Could you check a few things on this model? Use its own coordinates, in mm. A direction names the side the tool comes from. Give positions to 0.01 mm unless a question says otherwise; leave off trailing zeros. Loops run counter-clockwise (first coordinate to the right, second up) from the corner with the lowest first, then second, coordinate; pieces in that order, holes last. Notation, with made-up numbers: M -16.75,-33 L 18.25,-33 A24 ccw 18.25,0 Z; hole C 40,5.5 d11. An arc over 180 degrees is marked long. Use CSV: the item, a comma, the result in double quotes.
```python
from build123d import *

# Parameters (mm, degrees)
SKETCH1_W               = 240
SKETCH1_H               = 300
BOSS_EXTRUDE1_DEPTH     = 80
SHELL1_T                = -11
SKETCH4_R               = 1.5
CUT_EXTRUDE2_DEPTH      = 209.086520467
MIRROR2_COPY_1_SKETCH_R = 1.5
MIRROR2_COPY_1_DEPTH    = 209.086520467
SKETCH16_W              = 25
SKETCH16_H              = 8
CUT_EXTRUDE9_DEPTH      = 333.866339542
SKETCH18_W              = 71.1
SKETCH18_H              = 45
SKETCH18_W_2            = 72.7
CUT_EXTRUDE10_DEPTH     = 295.108823397
SKETCH19_W              = 71.1
SKETCH19_H              = 7.810897368
SKETCH19_W_2            = 72.674166019
CUT_EXTRUDE11_DEPTH     = 295.108823397
CUT_EXTRUDE12_DEPTH     = 15


with BuildPart() as part:
    # Sketch1 → Boss-Extrude1 (new body)
    with BuildSketch(Plane(origin=(0, 0, 0), x_dir=(1, 0, 0), z_dir=(0, 1, 0))):
        Rectangle(SKETCH1_W, SKETCH1_H)
    extrude(amount=BOSS_EXTRUDE1_DEPTH)

    # Shell1
    shell1_openings = [part.faces().sort_by_distance(p)[0] for p in [
        (0, 80, 0),
        (0, 0, 0),
    ]]
    offset(amount=SHELL1_T, openings=shell1_openings, kind=Kind.INTERSECTION)

    # Sketch4 → Cut-Extrude2 (cut, through all)
    with BuildSketch(Plane(origin=(0, 80, 0), x_dir=(1, 0, 0), z_dir=(0, 1, 0))):
        with Locations(Location((-112.5, 142.5, 0), (0, 0, 270))):
            Circle(SKETCH4_R)
    cut_extrude2 = extrude(amount=-CUT_EXTRUDE2_DEPTH, mode=Mode.SUBTRACT)

    # Mirror1: Cut-Extrude2 across plane
    add(cut_extrude2.mirror(Plane(origin=(0, 0, 0), x_dir=(0, 0, 1), z_dir=(1, 0, 0))), mode=Mode.SUBTRACT)

    # Mirror2: Cut-Extrude2 across plane
    add(cut_extrude2.mirror(Plane.XY), mode=Mode.SUBTRACT)

    # Mirror2 copy 1 sketch → Mirror2 copy 1 (cut, through all)
    with BuildSketch(Plane(origin=(0, 80, 0), x_dir=(-1, 0, 0), z_dir=(0, 1, 0))):
        with Locations(Location((-112.5, 142.5, 0), (0, 0, 270))):
            Circle(MIRROR2_COPY_1_SKETCH_R)
    extrude(amount=-MIRROR2_COPY_1_DEPTH, mode=Mode.SUBTRACT)

    # Sketch16 → Cut-Extrude9 (cut, through all)
    with BuildSketch(Plane.XY.offset(150)):
        with Locations((-67.5, 4)):
            Rectangle(SKETCH16_W, SKETCH16_H)
    cut_extrude9 = extrude(amount=-CUT_EXTRUDE9_DEPTH, mode=Mode.SUBTRACT)

    # Mirror3: Cut-Extrude9 across plane
    add(cut_extrude9.mirror(Plane(origin=(0, 0, 0), x_dir=(0, 0, 1), z_dir=(1, 0, 0))), mode=Mode.SUBTRACT)

    # Sketch18 → Cut-Extrude10 (cut, through all)
    with BuildSketch(Plane(origin=(120, 0, 0), x_dir=(0, 0, -1), z_dir=(1, 0, 0))):
        with Locations((-82.48, 22.5)):
            Rectangle(SKETCH18_W, SKETCH18_H)
        with Locations((23.65, 22.5)):
            Rectangle(SKETCH18_W_2, SKETCH18_H)
    extrude(amount=-CUT_EXTRUDE10_DEPTH, mode=Mode.SUBTRACT)

    # Sketch19 → Cut-Extrude11 (cut, through all)
    with BuildSketch(Plane(origin=(120, 0, 0), x_dir=(0, 0, -1), z_dir=(1, 0, 0))):
        with Locations((-82.48, 48.905448684)):
            Rectangle(SKETCH19_W, SKETCH19_H)
        with Locations((23.637083009, 48.905448684)):
            Rectangle(SKETCH19_W_2, SKETCH19_H)
    extrude(amount=-CUT_EXTRUDE11_DEPTH, mode=Mode.SUBTRACT)

    # Sketch22 → Cut-Extrude12 (cut)
    with BuildSketch(Plane(origin=(0, 0, -150), x_dir=(-1, 0, 0), z_dir=(0, 0, -1))):
        Polygon((-28.041535061, 0), (30, 0), (30, 72.971763315), (-30.071746562, 72.971763315), align=None)
    extrude(amount=-CUT_EXTRUDE12_DEPTH, mode=Mode.SUBTRACT)


solid = part.part
```
1. I'm going to push flat-ended pins straight in: pin 1 Ø9 at (x, z) = (113.5, 85.5) entering from -Y; pin 2 Ø9 at (x, z) = (-67.5, 143) entering from -Y. Where does each tip first touch, or does it pass through?
Outcome:
pin 1,"y = 52.81"
pin 2,"y = 8"
2. If we mould it in two halves opening along Z, with no side actions, what happens to faces 1 (the face through (115, 26, 118.03)), 2 (the face through (114, 0, 30)), 3 (the face through (-114, 26, 46.93))? For each: +Z half, -Z half, draft (parallel to the pull), parting line (faces both ways), or undercut.
Outcome:
face 1,"undercut"
face 2,"draft"
face 3,"undercut"
3. I want a section at B-B, the plane y = 36. Give the number of separate pieces and of enclosed holes in the cut face, then the cut area to 3 significant figures.
Outcome:
separate pieces,"5"
enclosed holes,"4"
area,"7,550 mm2"
4. Which directions (+Z, -Z, +X, -X, +Y, -Y) give clear straight access to the entire face, cutting with the end or side of a thin tool? Please do faces 4 (the face through (-80, 4, -144)), 5 (the face through (115, 52.811, 83)), 6 (the face through (109, 57, 2)), 7 (the face through (-109.2, 0, -115.6)).
Outcome:
face 4,"+Z, -Z, -Y"
face 5,"+X, -X, -Y"
face 6,"+Y, -Y"
face 7,"+Z, -Z, +X, -X, -Y"
5. I want a section at C-C, the plane z = 90.5. List the corners of the cut face in (x, y) for me, then the cut area to 3 significant figures.
Outcome:
outline,"M -120,52.81 L -109,52.81 L -109,80 L -120,80 Z; M 109,52.81 L 120,52.81 L 120,80 L 109,80 Z"
area,"598 mm2"
6. Please list where these lines run through material, in increasing order: line 1 (X direction, y = 18, z = 142.5); line 2 (Z direction, x = -112.5, y = 38.5); line 3 (X direction, y = 28, z = -134).
Outcome:
line 1,"-120 to -114, -111 to 111, 114 to 120"
line 2,"-150 to -144, -141 to -60, 12.7 to 46.93, 118.03 to 141, 144 to 150"
line 3,"-120 to -109, 109 to 120"
7. I want a section at A-A, the plane x = 101.5. List the corners of the cut face in (y, z) for me, then the cut area to 3 significant figures.
Outcome:
outline,"M 0,-150 L 80,-150 L 80,-139 L 0,-139 Z; M 0,139 L 80,139 L 80,150 L 0,150 Z"
area,"1,760 mm2"
